Input: part model. Units: mm. Frame: model coordinates. A direction names the side the tool comes from. Coordinates: 2 decimals unless noted, no trailing zeros. Order: outer loops, then holes, each group sorted by start corner. A loop starts at its lowest first (then second) coordinate and runs counter-clockwise, first axis right, second up. Notation, with made-up numbers: (-16.5, -15) - (26.5, -15) arc R28 ccw to (26.5, 14) - close; hole circle Ø7 at (49, 7.25). An arc over 180 degrees is marked (long way). One line per question, with ' | ' between items. Start each with the question number.
```python
from build123d import *

# Parameters (mm, degrees)
F0_W     = 19.05
F0_H     = 38.1
F0_H_2   = 19.05
F0_W_2   = 38.1
F1_DEPTH = 19.05
F2_W     = 38.1
F2_H     = 19.05
F2_W_2   = 19.05
F3_DEPTH = 19.05
F4_W     = 19.05
F4_H     = 38.1
F5_DEPTH = 19.05
F6_DEPTH = 25.4


with BuildPart() as f1:
    # F0 (on Right) → F1 (new body)
    with BuildSketch(Plane.YZ):
        with Locations((-9.525, 38.1)):
            Rectangle(F0_W, F0_H)
        with Locations((-9.525, 9.525)):
            Rectangle(F0_W, F0_H_2)
        with Locations((-38.1, 9.525)):
            Rectangle(F0_W_2, F0_H_2)
    extrude(amount=F1_DEPTH)

    # F2 (on face) → F3 (join)
    with BuildSketch(Plane(origin=(0, 0, 0), x_dir=(0, -1, 0), z_dir=(-1, 0, 0))):
        with Locations((38.1, 9.525)):
            Rectangle(F2_W, F2_H)
        with Locations((9.525, 9.525)):
            Rectangle(F2_W_2, F2_H)
    extrude(amount=F3_DEPTH)

    # F4 (on face) → F5 (join)
    with BuildSketch(Plane(origin=(-19.05, 0, 0), x_dir=(0, -1, 0), z_dir=(-1, 0, 0))):
        with Locations((9.525, 38.1)):
            Rectangle(F4_W, F4_H)
        Polygon((19.05, 19.05), (0, 19.05), (0, 0), (57.15, 0), (57.15, 19.05), align=None)
    extrude(amount=F5_DEPTH)

    # F5_face (on face) → F6 (join)
    with BuildSketch(Plane(origin=(-9.525, 0, 25.853571), x_dir=(-1, 0, 0), z_dir=(0, 1, 0))):
        Polygon((-9.525, 31.296429), (-28.575, 31.296429), (-28.575, -25.853571), (28.575, -25.853571), (28.575, 31.296429), (9.525, 31.296429), (9.525, -6.803571), (-9.525, -6.803571), align=None)
    extrude(amount=F6_DEPTH)


solid = f1.part
```
(1) Section C-C (x = 7). Output: boundary loops of the cut face in (y, z).
(2) Material intervals for line 1 along Y through (x, z) = (1.5, 39.5); line 2 along X through (y, z) = (-12.5, 25); line 3 along Z through (x, y) = (-8, -41), sorted ascending. Write a range as from..to.
(3) Section A-A (z = 21). Output: boundary loops of the cut face in (x, y), then the cut area to 3 significant figures.
(4) Section D-D (y = -20.5). Output: boundary loops of the cut face in (x, z).
(5) Pin query (flat end, axial travel): pin 1 (15 mm diameter, centred on x = 6.5, z = 30.5, fed in from -Y); pin 2 (2 mm diameter, centred on x = -9, y = -29.5, fed in from +Z). Return the tip coordinate at first contact, or that it passes through.
(6) Reachability of faces 4 (the face through (-28, -19.05, 38)), 5 (the face through (0, 3, 38)), 6 (the face through (19.05, -7, 23)) from +Z, -Z, +X, -X, +Y, -Y: full face, straight path, thin tool, end or side. Return the list, or none.
(7) Section B-B (y = 0). Output: boundary loops of the cut face in (x, z), then the cut area to 3 significant figures.
(8) Draft query along X for faces 1 (the face through (-10, -26, 19.05)), 2 (the face through (-38.1, -7, 22)), 3 (the face through (9, 3, 57.15)). Return one class per face: +X half, -X half, draft (parallel to the pull), parting line (faces both ways), or undercut.
Worked answers:
1) outline: (-57.15, 0) - (25.4, 0) - (25.4, 57.15) - (-19.05, 57.15) - (-19.05, 19.05) - (-57.15, 19.05) - close
2) line 1: y = -19.05..25.4 | line 2: x = -38.1..-19.05, 0..19.05 | line 3: z = 0..19.05
3) outline: (-38.1, -19.05) - (-19.05, -19.05) - (-19.05, 25.4) - (-38.1, 25.4) - close; (0, -19.05) - (19.05, -19.05) - (19.05, 25.4) - (0, 25.4) - close | area: 1,690 mm²
4) outline: (-38.1, 0) - (19.05, 0) - (19.05, 19.05) - (-38.1, 19.05) - close
5) pin 1: stops at y = -19.05 | pin 2: stops at z = 19.05
6) face 4: +Z, +X, -X, -Y | face 5: +Z, +Y, -Y | face 6: +Z, -Z, +X, +Y, -Y
7) outline: (-38.1, 0) - (19.05, 0) - (19.05, 57.15) - (0, 57.15) - (0, 19.05) - (-19.05, 19.05) - (-19.05, 57.15) - (-38.1, 57.15) - close | area: 2,540 mm²
8) face 1: undercut | face 2: -X half | face 3: draft
